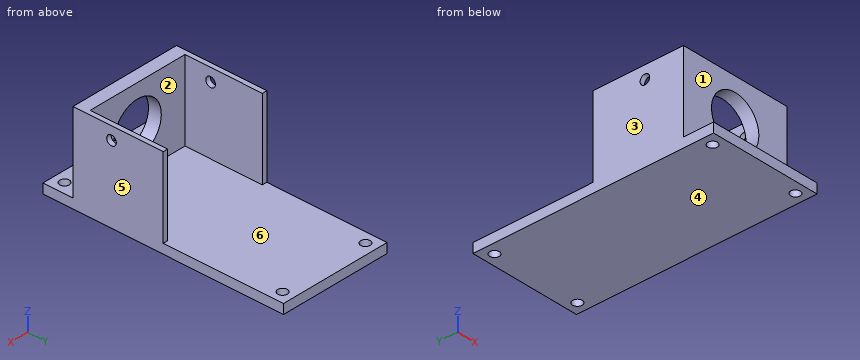
from build123d import *

# Parameters (mm, degrees)
SKETCH1_W           = 35
SKETCH1_H           = 75
BOSS_EXTRUDE1_DEPTH = 3
SKETCH2_R           = 1.5
SIDE_HOLES_DEPTH    = 13
SKETCH3_W           = 32
SKETCH3_H           = 4
BOSS_EXTRUDE2_DEPTH = 25
SKETCH4_R           = 8
CUT_EXTRUDE2_DEPTH  = 5
SKETCH5_W           = 25
SKETCH5_H           = 28.130280997
BOSS_EXTRUDE3_DEPTH = 1.5
SKETCH6_W           = 25
SKETCH6_H           = 28.130280997
BOSS_EXTRUDE4_DEPTH = 1.5
SKETCH7_R           = 1.5
CUT_EXTRUDE3_DEPTH  = 59.440140315


with BuildPart() as part:
    # Sketch1 → Boss-Extrude1 (new body)
    with BuildSketch(Plane.XY):
        Rectangle(SKETCH1_W, SKETCH1_H)
    extrude(amount=BOSS_EXTRUDE1_DEPTH)

    # Sketch2 → side holes (cut)
    with BuildSketch(Plane.XY.offset(3)):
        with Locations((14, 34)):
            Circle(SKETCH2_R)
        with Locations((-14, 34)):
            Circle(SKETCH2_R)
        with Locations((14, -34)):
            Circle(SKETCH2_R)
        with Locations((-14, -34)):
            Circle(SKETCH2_R)
    extrude(amount=-SIDE_HOLES_DEPTH, mode=Mode.SUBTRACT)

    # Sketch3 → Boss-Extrude2 (add)
    with BuildSketch(Plane.XY.offset(3)):
        with Locations((0, -26.130280997)):
            Rectangle(SKETCH3_W, SKETCH3_H)
    extrude(amount=BOSS_EXTRUDE2_DEPTH)

    # Sketch4 → Cut-Extrude2 (cut)
    with BuildSketch(Plane.XZ.offset(28.130280997)):
        with Locations(Location((0, 15.5, 0), (0, 0, 270))):
            Circle(SKETCH4_R)
    extrude(amount=-CUT_EXTRUDE2_DEPTH, mode=Mode.SUBTRACT)

    # Sketch5 → Boss-Extrude3 (add)
    with BuildSketch(Plane.ZY.offset(16)):
        with Locations((15.5, -14.065140499)):
            Rectangle(SKETCH5_W, SKETCH5_H)
    extrude(amount=BOSS_EXTRUDE3_DEPTH)

    # Sketch6 → Boss-Extrude4 (add)
    with BuildSketch(Plane(origin=(16, 0, 0), x_dir=(0, 0, -1), z_dir=(1, 0, 0))):
        with Locations((-15.5, -14.065140499)):
            Rectangle(SKETCH6_W, SKETCH6_H)
    extrude(amount=BOSS_EXTRUDE4_DEPTH)

    # Sketch7 → Cut-Extrude3 (cut, through all)
    with BuildSketch(Plane(origin=(17.5, 0, 0), x_dir=(0, 0, -1), z_dir=(1, 0, 0))):
        with Locations((-24, -16.130280997)):
            Circle(SKETCH7_R)
    extrude(amount=-CUT_EXTRUDE3_DEPTH, mode=Mode.SUBTRACT)


solid = part.part
The model under review builds one solid part; all positions refer to its coordinate system, in mm. Face numbers are marked on the shaded views. A direction names the side the tool comes from. Coordinates: 2 decimals unless noted, no trailing zeros. Write each loop counter-clockwise with the first axis right and the second up, starting at its lowest first coordinate (ties: lowest second). Pieces come first, ordered by that corner, then holes. Notation, with made-up numbers: M 45.5,-24.5 L 90.5,-24.5 A18 cw 90.5,-9.5 Z; hole C 62.5,57 d7. An arc over 180 degrees is marked long. Put each result on its own line as item: value.
1) Add section B-B on x = 14. Give the boundary of the cut face in (y, z).
Computed:
outline: M -37.5,0 L -35.5,0 L -35.5,3 L -37.5,3 Z; M -32.5,0 L 32.5,0 L 32.5,3 L -24.13,3 L -24.13,28 L -28.13,28 L -28.13,3 L -32.5,3 Z; M 35.5,0 L 37.5,0 L 37.5,3 L 35.5,3 Z
2) Clearance check with flat-ended pins moving along their axes: pin 1 Ø2.5 at (x, y) = (-14, -34) entering from +Z; pin 2 Ø0.8 at (x, z) = (16.5, 16) entering from +Y; pin 3 Ø4 at (x, y) = (14, 34) entering from +Z. State where each tip first meets the part, or that it passes through.
Computed:
pin 1: passes through
pin 2: stops at y = 0
pin 3: stops at z = 3
3) Add section D-D on x = 1.5. Give the boundary of the cut face in (y, z).
Computed:
outline: M -37.5,0 L 37.5,0 L 37.5,3 L -24.13,3 L -24.13,7.64 L -28.13,7.64 L -28.13,3 L -37.5,3 Z; M -28.13,23.36 L -24.13,23.36 L -24.13,28 L -28.13,28 Z
4) For the marked faces 1, 2 and 3, list the 3-axis set-ups (+Z, -Z, +X, -X, +Y, -Y) from which the entire face can be reached by the end or side of a thin tool; tool diameter is ignored.
Computed:
face 1: +Z, +X, -X, -Y
face 2: +Z, +Y
face 3: +Z, -Z, -X, +Y, -Y
5) Add section A-A on y = -34. Give the boundary of the cut face in (x, z), then the cut area to 3 significant figures.
Computed:
outline: M -17.5,0 L -15.5,0 L -15.5,3 L -17.5,3 Z; M -12.5,0 L 12.5,0 L 12.5,3 L -12.5,3 Z; M 15.5,0 L 17.5,0 L 17.5,3 L 15.5,3 Z
area: 87.0 mm2
6) Wall thickness on probe 1 along Y at (x, z) = (-14, 2.1); probe 2 along X at (y, z) = (-2, 14.5); probe 3 along X at (y, z) = (-26.25, 15.5): over which ranges is each line inside the solid? List them lowest first. Write a range as [from, to].
Computed:
probe 1: y = [-37.5, -35.5], [-32.5, 32.5], [35.5, 37.5]
probe 2: x = [-17.5, -16], [16, 17.5]
probe 3: x = [-17.5, -8], [8, 17.5]
7) Draft analysis for pull direction X (two halves, no side actions). For the marked faces 4, 5 and 6, state which applies: released by +X, released by -X, zero draft, split by the parting line, or undercut.
Computed:
face 4: zero draft
face 5: released by +X
face 6: undercut
8) Add section C-C on z = 15.5. Give the boundary of the cut face in (x, y).
Computed:
outline: M -17.5,-28.13 L -8,-28.13 L -8,-24.13 L -16,-24.13 L -16,0 L -17.5,0 Z; M 8,-28.13 L 17.5,-28.13 L 17.5,0 L 16,0 L 16,-24.13 L 8,-24.13 Z
